Geometry check sheet. Reference: the model listing, model coordinates, mm. A direction names the side the tool comes from. Coordinates: 2 decimals unless noted, no trailing zeros. Write each loop counter-clockwise with the first axis right and the second up, starting at its lowest first coordinate (ties: lowest second). Pieces come first, ordered by that corner, then holes. Notation, with made-up numbers: (66, -4) - (96, -4) arc R28 ccw to (96, 31) - close; hole circle Ø11 at (50, -1). An arc over 180 degrees is marked (long way). Answer as a JSON object with one key per item and string values. Group by question number.
from build123d import *

# Parameters (mm, degrees)
SKETCH001_R  = 0.5
PAD001_DEPTH = 3.5
SKETCH_W     = 11.5
SKETCH_H     = 11.5
PAD_DEPTH    = 9.6
FILLET_R     = 1


with BuildPart() as pad001:
    # Sketch001 → Pad001 (new body)
    with BuildSketch(Plane.XY.offset(0.5)):
        Circle(SKETCH001_R)
        with Locations((6, 6)):
            Circle(SKETCH001_R)
    extrude(amount=-PAD001_DEPTH)


with BuildPart() as obj1:
    # Sketch → Pad (new body)
    with BuildSketch(Plane.XY.offset(0.1)):
        with Locations((3, 3)):
            Rectangle(SKETCH_W, SKETCH_H)
    extrude(amount=PAD_DEPTH)

    # Fillet
    fillet_edges = [obj1.edges().sort_by_distance(p)[0] for p in [
        (8.75, -2.75, 4.9),
        (8.75, 8.75, 4.9),
        (-2.75, -2.75, 4.9),
        (-2.75, 8.75, 4.9),
    ]]
    fillet(fillet_edges, radius=FILLET_R)

    # obj1: union Pad001
    add(pad001.part)


solid = obj1.part
(1) Section check B-B (x = 6). Record the cut outline in (y, z), and give its area (4 significant figures).
(2) Section check C-C (z = -1). Record the cut outline in (x, y).
(3) Section check D-D (x = 3.25). Record the cut outline in (y, z).
(4) Section check A-A (y = 0). Record the cut outline in (x, z).
(5) Set-up check for faces 1 (the face through (-0.108, -0.488, -1.428)), 2 (the face through (8.465, 8.449, 4.967)): record each of +Z, -Z, +X, -X, +Y, -Y from which the full face is reachable in a straight line by a thin tool's end or side.
(6) Gauge pin test, flat end, axial feed: pin 1 (1 mm diameter, centred on x = 7, y = 7, fed in from -Z). Record the tip position at first contact, or that the pin passes through.
(7) Material ranges on L1, parallel to Z at x = 0.25, y = 6.5; L2, parallel to Y at x = 0, z = -1.75; L3, parallel to Y at x = -2, z = 8.25, recorded low to high. Write a range as [from, to].
Conclusion:
{
 "1": {"outline": "(-2.75, 0.1) - (5.5, 0.1) - (5.5, -3) - (6.5, -3) - (6.5, 0.1) - (8.75, 0.1) - (8.75, 9.7) - (-2.75, 9.7) - close", "area": "113.5 mm^2"},
 "2": {"outline": "circle Ø1 at (0, 0); circle Ø1 at (6, 6)"},
 "3": {"outline": "(-2.75, 0.1) - (8.75, 0.1) - (8.75, 9.7) - (-2.75, 9.7) - close"},
 "4": {"outline": "(-2.75, 0.1) - (-0.5, 0.1) - (-0.5, -3) - (0.5, -3) - (0.5, 0.1) - (8.75, 0.1) - (8.75, 9.7) - (-2.75, 9.7) - close"},
 "5": {"face 1": "-Z", "face 2": "+Z, -Z, +X, +Y"},
 "6": {"pin 1": "stops at z = 0.1"},
 "7": {"L1": "z = [0.1, 9.7]", "L2": "y = [-0.5, 0.5]", "L3": "y = [-2.72, 8.72]"}
}
